Autodesk Inventor part; units mm, degrees
ref_plane "YZ Plane" through (0, 0, 0) normal (1, 0, 0) x (0, 1, 0)
ref_plane "XZ Plane" through (0, 0, 0) normal (0, 1, 0) x (-1, 0, 0)
ref_plane "XY Plane" through (0, 0, 0) normal (0, 0, 1) x (1, 0, 0)
sketch "Sketch1" plane through (0, 0, 0) normal (0, 0, 1) x (1, 0, 0)
  line L0 (-30, -7.5) -> (30, -7.5)
  line L1 (30, -7.5) -> (30, 7.5)
  line L2 (30, 7.5) -> (-30, 7.5)
  line L3 (-30, 7.5) -> (-30, -7.5)
  line L4 (-30, -7.5) -> (30, 7.5) construction
  line L5 (30, -7.5) -> (-30, 7.5) construction
  line L6 (30, 7.5) -> (25, 7.5) construction
  line L7 (-30, 7.5) -> (-25, 7.5) construction
  point P0 (0, 0)
  dimension "d0" = 60
  dimension "d1" = 15
extrude "Block" add sketch "Sketch1" along normal blind 60
sketch "Sketch2" plane through (30, -7.5, 0) normal (1, 0, 0) x (0, 0, -1)
  line L0 (0, 15) -> (-60, 15)
  line L1 (-30, 15) -> (-12.75, 15)
  line L2 (-30, 15) -> (-47.25, 15)
  line L3 (-30, 15) -> (-30, 6.1) construction
  line L4 (-30, 6.1) -> (-6.75, 6.1)
  line L5 (-30, 6.1) -> (-53.25, 6.1)
  line L6 (-53.25, 6.1) -> (-53.25, 8.1)
  line L7 (-6.75, 6.1) -> (-6.75, 8.1)
  line L8 (-6.75, 8.1) -> (-12.75, 15)
  line L9 (-53.25, 8.1) -> (-47.25, 15)
  point P0 (0, 7.5)
  dimension "d17" = 17.25
  dimension "d18" = 17.25
  dimension "d19" = 8.9
  dimension "d20" = 23.25
  dimension "d21" = 23.25
  dimension "d22" = 2
  dimension "d23" = 2
extrude "Tripod Slot" cut sketch "Sketch2" against normal blind 60
hole "Hole1" at (0, -1.4, 30) direction (0, -1, 0) diameter 22.5 end through all
sketch "Sketch4" plane through (0, 0, 0) normal (0, 0, -1) x (-1, 0, 0)
  line L0 (-30, 7.5) -> (30, 7.5)
  line L1 (12.7, 7.5) -> (-12.7, 7.5)
  line L2 (-12.7, 7.5) -> (-12.7, -7.5)
  line L3 (30, -7.5) -> (-30, -7.5)
  line L4 (-12.7, -7.5) -> (12.7, -7.5)
  line L5 (12.7, -7.5) -> (12.7, 7.5)
  point P0 (0, 1.5)
  dimension "d64" = 25.4
  dimension "d96" = 17.3
  dimension "d97" = 9
  dimension "d98" = 12.7
extrude "Extrusion4" add sketch "Sketch4" along normal blind 49.5
sketch "Sketch5" plane through (-30, 7.5, 12.75) normal (0, 1, 0) x (1, 0, 0)
  line L0 (60, -34.5) -> (60, 0)
  line L1 (17.3, 62.25) -> (42.7, 62.25)
  line L2 (17.3, 62.25) -> (42.7, 62.25)
  line L3 (42.7, 62.25) -> (42.7, 39.75)
  line L4 (42.7, 39.75) -> (17.3, 39.75)
  line L5 (17.3, 39.75) -> (17.3, 62.25)
  line L6 (42.7, 39.75) -> (17.3, 62.25) construction
  circle A0 centre (30, 51) radius 1.5
  point P0 (30, 12.75)
  dimension "d67" = 22.5
  dimension "d68" = 3
  dimension "d99" = 131.535
extrude "Extrusion5" add sketch "Sketch5" along normal blind 40
sketch "Sketch6" plane through (0, 0, -49.5) normal (0, 0, -1) x (-1, 0, 0)
  line L0 (0, 0) -> (0, 47.5) construction
  circle A0 centre (0, 37.5) radius 2.5
  line L1 (-12.7, 47.5) -> (12.7, 47.5) construction
  line L2 (-12.7, 47.5) -> (12.7, 47.5) construction
  line L3 (12.7, 47.5) -> (0, 47.5) construction
  line L4 (0, 37.5) -> (0, 47.5) construction
  dimension "d60" = 5
  dimension "d61" = 10
extrude "Extrusion6" cut sketch "Sketch6" against normal blind 31.75
fillet "Fillet4" radius 11 2 edges at (12.7, 47.5, -38.25) (-12.7, 47.5, -38.25)
fillet "Fillet5" radius 20 1 edges at (0, -7.5, -49.5)
fillet "Fillet6" radius 5 1 edges at (0, 7.5, -27)
fillet "Fillet10" radius 7.5 2 edges at (12.7, 0, 0) (-12.7, 0, 0)
fillet "Fillet11" radius 1.5 2 edges at (0, -7.5, 18.75) (0, -1.4, 18.75)
properties part number "InnerFrame"
Design review of the part built by this model. Coordinates are the model's own, in mm. A direction names the side the tool comes from. Coordinates: 2 decimals unless noted, no trailing zeros. Loops run counter-clockwise (first coordinate to the right, second up) from the corner with the lowest first, then second, coordinate; pieces in that order, holes last.
Q1. We need section B-B on y = 2. State the section outline as (x, z) points.
Reported:
outline: (-30, 0) - (-20.2, 0) arc R7.5 cw to (-12.7, -7.5) - (-12.7, -46.52) - (12.7, -46.52) - (12.7, -7.5) arc R7.5 cw to (20.2, 0) - (30, 0) - (30, 7.97) - (-30, 7.97) - close; (-30, 52.03) - (30, 52.03) - (30, 60) - (-30, 60) - close
Q2. We need section D-D on y = 23.5. State the section outline as (x, z) points.
Reported:
outline: (-12.7, -49.5) - (12.7, -49.5) - (12.7, -27) - (-12.7, -27) - close; hole circle Ø3 at (0, -38.25)
Q3. Tool access review of faces 1 (the face through (0, 30, -27)), 2 (the face through (9.563, 44.192, -38.092)), 3 (the face through (25, 0, 0)), 4 (the face through (7, -1.4, 19)), 5 (the face through (0, 0, 60)): name each direction out of +Z, -Z, +X, -X, +Y, -Y from which nothing blocks a thin tool from reaching the whole face with its end or side.
Reported:
face 1: +Z, +X, -X, +Y
face 2: +Z, -Z, +X, +Y
face 3: -Z, +X, +Y, -Y
face 4: +X, -X
face 5: +Z, +X, -X, +Y, -Y
Q4. To check wall thickness, follow line 1 (Z direction, x = 0, y = 27.5); line 2 (X direction, y = 14.75, z = -38.25); line 3 (Y direction, x = -24.5, z = 41.5). State the ranges of each line that lie inside material, in increasing order.
Reported:
line 1: z = -49.5 to -39.75, -36.75 to -27
line 2: x = -12.7 to -1.5, 1.5 to 12.7
line 3: y = -7.5 to -1.4
Q5. We need section A-A on z = 30. State the section outline as (x, y) points, and give its area (3 significant figures).
Reported:
outline: (-30, -7.5) - (-12.75, -7.5) arc R1.5 ccw to (-11.25, -6) - (-11.25, -2.9) arc R1.5 ccw to (-12.75, -1.4) - (-30, -1.4) - close; (11.25, -6) arc R1.5 ccw to (12.75, -7.5) - (30, -7.5) - (30, -1.4) - (12.75, -1.4) arc R1.5 ccw to (11.25, -2.9) - close
area: 227 mm2
Q6. For pin 1 (21 mm diameter, centred on y = 8.5, z = -28, fed in from +X); pin 2 (10 mm diameter, centred on x = 4, z = 55.5, fed in from +Y); pin 3 (1.6 mm diameter, centred on x = -9.5, y = -0.5, fed in from -Z), all flat-tipped, find the tip position at first contact; note any pin that passes through.
Reported:
pin 1: stops at x = 12.7
pin 2: stops at y = 7.5
pin 3: stops at z = -45.35
Q7. We need section C-C on x = 0. State how many separate pieces and enclosed holes the cut face has, and give its area (3 significant figures).
Reported:
separate pieces: 4
enclosed holes: 0
area: 1,730 mm2
Q8. The part is to be moulded in two halves that separate along Z. For faces 6 (the face through (-25, 0, 0)), 7 (the face through (-0.195, 43.444, -36.763)), 8 (the face through (-12.7, 14, -33)), 9 (the face through (-0.18, 9, -25.57)), say which applies: +Z half, -Z half, draft (parallel to the pull), parting line (faces both ways), or undercut.
Reported:
face 6: -Z half
face 7: undercut
face 8: draft
face 9: +Z half
